from build123d import *

# Parameters (mm, degrees)
F0_W     = 72
F0_H     = 163
F1_DEPTH = 5
F2_W     = 30
F2_H     = 26
F2_R     = 7.5
F3_DEPTH = 25
F4_R     = 10.8639610307
F5_R     = 5.3112698372


with BuildPart() as f1:
    # F0 (on Top) → F1 (new body)
    with BuildSketch(Plane.XY):
        with Locations((-8.3418504, 45.0741375387)):
            Rectangle(F0_W, F0_H)
    extrude(amount=-F1_DEPTH)

    # F2 (on face) → F3 (cut)
    with BuildSketch(Plane.XY):
        with Locations((12.6581496, 96.5741375387)):
            Rectangle(F2_W, F2_H)
        with Locations((-29.3418504, 96.5741375387)):
            Rectangle(F2_W, F2_H)
        with Locations((12.6581496, 68.5741375387)):
            Circle(F2_R)
        with Locations((-29.3418504, 68.5741375387)):
            Circle(F2_R)
        with Locations((-8.3418504, 38.5741375387)):
            Circle(F2_R)
        with Locations((-29.3418504, -21.4258624613)):
            Circle(F2_R)
        with Locations((12.6581496, -21.4258624613)):
            Circle(F2_R)
        with Locations((12.6581496, 38.5741375387)):
            Circle(F2_R)
        with Locations((-8.3418504, 68.5741375387)):
            Circle(F2_R)
        with Locations((-29.3418504, 38.5741375387)):
            Circle(F2_R)
        with Locations((-8.3418507129, -21.4258624613)):
            Circle(F2_R)
        with Locations((-29.3418504, 8.5741375387)):
            Circle(F2_R)
        with Locations((12.6581492871, 8.5741375387)):
            Circle(F2_R)
        with Locations((-8.3418507129, 8.5741375387)):
            Circle(F2_R)
    extrude(amount=-F3_DEPTH, mode=Mode.SUBTRACT)

    # F4
    f4_edges = [f1.edges().sort_by_distance(p)[0] for p in [
        (-2.34185, 109.574138, -2.5),
        (-2.34185, 83.574138, -2.5),
        (-14.34185, 83.574138, -2.5),
        (-14.34185, 109.574138, -2.5),
    ]]
    fillet(f4_edges, radius=F4_R)

    # F5
    f5_edges = [f1.edges().sort_by_distance(p)[0] for p in [
        (27.65815, 126.574138, -2.5),
        (-44.34185, 126.574138, -2.5),
        (-44.34185, 109.574138, -2.5),
        (-44.34185, 83.574138, -2.5),
        (27.65815, 109.574138, -2.5),
        (27.65815, 83.574138, -2.5),
        (-44.34185, -36.425862, -2.5),
        (27.65815, -36.425862, -2.5),
    ]]
    fillet(f5_edges, radius=F5_R)


solid = f1.part
CAD build for the part. Positions are in the model's coordinates, mm. A direction names the side the tool comes from. Give positions to 0.01 mm unless a question says otherwise; leave off trailing zeros. Loops run counter-clockwise (first coordinate to the right, second up) from the corner with the lowest first, then second, coordinate; pieces in that order, holes last. Notation, with made-up numbers: M 13.25,-23 L 40.25,-23 A18 ccw 40.25,2 Z; hole C 47.5,-37.75 d3. An arc over 180 degrees is marked long. Answer in a Markdown table with one row per item. Add a question column.
Item 1: Tool access for faces 1 (the face through (-14.342, 97, -2)), 2 (the face through (-34.87, 43.64, -2.46)), 3 (the face through (0.756, 86.841, -2.535)): list every direction of +Z, -Z, +X, -X, +Y, -Y with a clear straight run to the whole face (end or side of a thin tool).
Item 2: Band-saw the part on B-B on x = -18. Give the cut face in (y, z), then the cut area to 3 significant figures.
Item 3: Drop flat-ended pins along their axis: P1, Ø13.5, axis at x = -29.34, y = 68.57, coming from the +Z side (1 decimal); P2, Ø19.5, axis at x = 12.66, y = 68.57, coming from the +Z side; P3, Ø2, axis at y = 96, z = -2, coming from the +X side. Give the stop position or say it passes through.
Item 4: Band-saw the part on C-C on y = 12. Give the cut face in (x, z), then the cut area to 3 significant figures.
Item 5: Mould opens along Y. For faces 4 (the face through (-44.342, 118, -2)), 5 (the face through (-42.827, 124.977, -2.535)), 6 (the face through (11.68, 76.01, -2.46)) say: +Y half, -Y half, draft (parallel to the pull), parting line (faces both ways), or undercut.
Item 6: Probe probe 1 along X at (y, z) = (39, -2.6); probe 2 along X at (y, z) = (37, -1.1); probe 3 along Y at (x, z) = (-32, -2). List the from-to ranges inside material, lowest first.
Item 7: Band-saw the part on D-D on x = -4. Give the cut face in (y, z), then the cut area to 3 significant figures.
Item 8: Band-saw the part on A-A on x = -32. Give the cut face in (y, z).
Reply:
| question | item | result |
|---|---|---|
| 1 | face 1 | +Z, -Z, -X |
| 1 | face 2 | +Z, -Z |
| 1 | face 3 | +Z, -Z, +X |
| 2 | outline | M -36.43,-5 L 86.31,-5 L 86.31,0 L -36.43,0 Z; M 106.84,-5 L 126.57,-5 L 126.57,0 L 106.84,0 Z |
| 2 | area | 712 mm^2 |
| 3 | P1 | passes through |
| 3 | P2 | stops at z = 0 |
| 3 | P3 | stops at x = -2.34 |
| 4 | outline | M -44.34,-5 L -36.01,-5 L -36.01,0 L -44.34,0 Z; M -22.67,-5 L -15.01,-5 L -15.01,0 L -22.67,0 Z; M -1.67,-5 L 5.99,-5 L 5.99,0 L -1.67,0 Z; M 19.33,-5 L 27.66,-5 L 27.66,0 L 19.33,0 Z |
| 4 | area | 160 mm^2 |
| 5 | face 4 | draft |
| 5 | face 5 | +Y half |
| 5 | face 6 | undercut |
| 6 | probe 1 | x = -44.34 to -36.83, -21.85 to -15.83, -0.85 to 5.17, 20.15 to 27.66 |
| 6 | probe 2 | x = -44.34 to -36.67, -22.01 to -15.67, -1.01 to 5.33, 19.99 to 27.66 |
| 6 | probe 3 | y = -36.43 to -28.44, -14.41 to 1.56, 15.59 to 31.56, 45.59 to 61.56, 75.59 to 83.57, 109.57 to 126.57 |
| 7 | outline | M -36.43,-5 L -27.54,-5 L -27.54,0 L -36.43,0 Z; M -15.31,-5 L 2.46,-5 L 2.46,0 L -15.31,0 Z; M 14.69,-5 L 32.46,-5 L 32.46,0 L 14.69,0 Z; M 44.69,-5 L 62.46,-5 L 62.46,0 L 44.69,0 Z; M 74.69,-5 L 126.57,-5 L 126.57,0 L 74.69,0 Z |
| 7 | area | 570 mm^2 |
| 8 | outline | M -36.43,-5 L -28.44,-5 L -28.44,0 L -36.43,0 Z; M -14.41,-5 L 1.56,-5 L 1.56,0 L -14.41,0 Z; M 15.59,-5 L 31.56,-5 L 31.56,0 L 15.59,0 Z; M 45.59,-5 L 61.56,-5 L 61.56,0 L 45.59,0 Z; M 75.59,-5 L 83.57,-5 L 83.57,0 L 75.59,0 Z; M 109.57,-5 L 126.57,-5 L 126.57,0 L 109.57,0 Z |
